Design review of the part built by this model. Coordinates are the model's own, in mm. Face numbers are marked on the shaded views. A direction names the side the tool comes from. Round coordinates to 2 decimals unless told otherwise and drop trailing zeros. Loops run counter-clockwise (first coordinate to the right, second up) from the corner with the lowest first, then second, coordinate; pieces in that order, holes last. Notation, with made-up numbers: M 66,42.5 L 102,42.5 A22 cw 102,60.5 Z; hole C 6,71 d6. An arc over 180 degrees is marked long. One line per item, written item: value. Start each with the question number.
Item 1: For line 1 along Z through (x, y) = (-1.75, 0); line 2 along Z through (x, y) = (1.75, 0); line 3 along Z through (x, y) = (-3.6, 0), list the stretches that pass through material, from the lowest coordinate up.
Item 2: We need section B-B (y = 0). Write out the cut boundary in (x, z).
Item 3: We need section C-C (y = 8). Write out the cut boundary in (x, z), then the cut area to 3 significant figures.
Item 4: We need section D-D (z = 11). Write out the cut boundary in (x, y).
Item 5: Mouldability with a two-part tool opening along Y and no side actions: class the marked faces 3, 4, 5 and 6 as released by +Y, released by -Y, zero draft, split by the parting line, or undercut.
Item 6: We need section A-A (z = 0). Write out the cut boundary in (x, y), then the cut area to 4 significant figures.
Item 7: For the marked faces 1 and 2, list the 3-axis set-ups (+Z, -Z, +X, -X, +Y, -Y) from which the entire face can be reached by the end or side of a thin tool; tool diameter is ignored.
Item 8: Clearance check with flat-ended pins moving along their axes: pin 1 (1.5 mm diameter, centred on x = -4, z = 10.5, fed in from -Y); pin 2 (2 mm diameter, centred on x = -3, z = 0.5, fed in from -Y); pin 3 (6.5 mm diameter, centred on y = 1.5, z = 11, fed in from +X); pin 4 (2 mm diameter, centred on y = -10.5, z = -10.5, fed in from +X). State where each tip first meets the part, or that it passes through.
from build123d import *

# Parameters (mm, degrees)
SKETCH1_W               = 5
SKETCH1_H               = 5
BOSS_EXTRUDE1_DEPTH     = 3
CUT_EXTRUDE1_DEPTH      = 8
CUT_EXTRUDE1_DEPTH_BACK = 6
CIRPATTERN1_COUNT       = 4


with BuildPart() as part:
    # Sketch1 → Revolve1 (revolve)
    with BuildSketch(Plane.XY):
        Polygon((-6, 25), (-6, 15), (6, 15), (6, 25), (5, 25), (5, 24.5), (-5, 24.5), (-5, 25), align=None)
        with Locations((-3.5, 2.5)):
            Rectangle(SKETCH1_W, SKETCH1_H)
    revolve(axis=Axis((0, 0, 0), (1, 0, 0)))

    # Sketch2 → Boss-Extrude1 (add)
    with BuildSketch(Plane(origin=(-6, 0, 0), x_dir=(0, 0, -1), z_dir=(1, 0, 0))):
        with BuildLine():
            Line((-3, 4), (-3, 14.696938457))
            ThreePointArc((-3, 14.696938457), (0, 15), (3, 14.696938457))
            Line((3, 14.696938457), (3, 4))
            ThreePointArc((3, 4), (0, 5), (-3, 4))
        make_face()
    boss_extrude1 = extrude(amount=BOSS_EXTRUDE1_DEPTH)

    # Sketch3 → Cut-Extrude1 (cut, two sides)
    with BuildSketch(Plane(origin=(-1, 0, 0), x_dir=(0, 0, -1), z_dir=(1, 0, 0))) as cut_extrude1_sk:
        with BuildLine():
            Line((-1.360147051, 1.6), (1.360147051, 1.6))
            ThreePointArc((1.360147051, 1.6), (0, -2.1), (-1.360147051, 1.6))
        make_face()
    extrude(amount=CUT_EXTRUDE1_DEPTH, mode=Mode.SUBTRACT)
    extrude(cut_extrude1_sk.sketch, amount=-CUT_EXTRUDE1_DEPTH_BACK, mode=Mode.SUBTRACT)

    # CirPattern1: Boss-Extrude1 ×4 about axis
    cirpattern1_axis = Axis((0, 0, 0), (1, 0, 0))
    for i in range(1, CIRPATTERN1_COUNT):
        add(boss_extrude1.rotate(cirpattern1_axis, i * 360 / CIRPATTERN1_COUNT))


solid = part.part
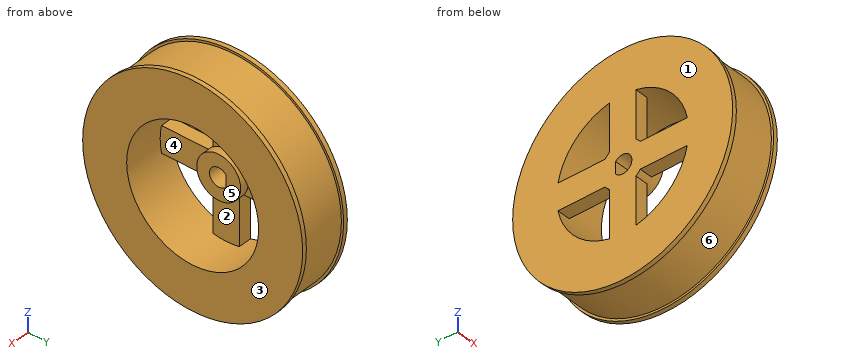
A:
1. line 1: -24.5 to -15, -5 to -2.1, 2.1 to 5, 15 to 24.5
1. line 2: -24.5 to -15, 15 to 24.5
1. line 3: -24.5 to -2.1, 2.1 to 24.5
2. outline: M -6,-25 L -5,-25 L -5,-24.5 L 5,-24.5 L 5,-25 L 6,-25 L 6,-15 L -3,-15 L -3,-5 L -1,-5 L -1,-2.1 L -6,-2.1 Z; M -6,2.1 L -1,2.1 L -1,5 L -3,5 L -3,15 L 6,15 L 6,25 L 5,25 L 5,24.5 L -5,24.5 L -5,25 L -6,25 Z
3. outline: M -6,-23.69 L -5,-23.69 L -5,-23.16 L 5,-23.16 L 5,-23.69 L 6,-23.69 L 6,-12.69 L -6,-12.69 Z; M -6,-3 L -3,-3 L -3,3 L -6,3 Z; M -6,12.69 L 6,12.69 L 6,23.69 L 5,23.69 L 5,23.16 L -5,23.16 L -5,23.69 L -6,23.69 Z
3. area: 271 mm2
4. outline: M -6,-22.45 L -5,-22.45 L -5,-21.89 L 5,-21.89 L 5,-22.45 L 6,-22.45 L 6,-10.2 L -6,-10.2 Z; M -6,-3 L -3,-3 L -3,3 L -6,3 Z; M -6,10.2 L 6,10.2 L 6,22.45 L 5,22.45 L 5,21.89 L -5,21.89 L -5,22.45 L -6,22.45 Z
5. face 3: zero draft
5. face 4: undercut
5. face 5: undercut
5. face 6: split by the parting line
6. outline: M -6,-25 L -5,-25 L -5,-24.5 L 5,-24.5 L 5,-25 L 6,-25 L 6,-15 L -3,-15 L -3,-5 L -1,-5 L -1,-2.1 L -6,-2.1 Z; M -6,1.6 L -1,1.6 L -1,5 L -3,5 L -3,15 L 6,15 L 6,25 L 5,25 L 5,24.5 L -5,24.5 L -5,25 L -6,25 Z
6. area: 321.5 mm2
7. face 1: +Z, -Z, -X, +Y, -Y
7. face 2: +X
8. pin 1: y = -22.48
8. pin 2: y = -24.5
8. pin 3: x = -3
8. pin 4: x = 6
